Verification items for the finished model (mm, model axes). Face numbers are marked on the shaded views. A direction names the side the tool comes from. Coordinates: 2 decimals unless noted, no trailing zeros. Order: outer loops, then holes, each group sorted by start corner. A loop starts at its lowest first (then second) coordinate and runs counter-clockwise, first axis right, second up. Notation, with made-up numbers: M 1,80.25 L 56,80.25 A22 ccw 56,115.25 Z; hole C 21.25,5 d7. An arc over 180 degrees is marked long. Answer as a JSON object with one key per item and string values. Group by question number.
(1) Access from +Z, -Z, +X, -X, +Y, -Y to the whole of each face (thin tool, end or side, straight path). Record for the marked faces 5 and 6.
(2) Material ranges on line 1 (Z direction, x = 13.1, y = -3.75); line 2 (Z direction, x = -3, y = -6); line 3 (X direction, y = -8.75, z = 31.5), recorded low to high.
(3) Gauge pin test, flat ends, axial feed: pin 1 Ø1.5 at (x, z) = (11, 37) entering from -Y; pin 2 Ø5 at (x, z) = (13.1, 33.2) entering from +Y. Record the tip position at first contact, or that the pin passes through.
(4) Cross-section at A-A (z = 33.2). Enter the section's corners in (x, y).
(5) Cross-section at B-B (y = -1.25). Count the separate pieces of the cut face and the enclosed holes in it, plus the area to 3 significant figures.
(6) Mould release check, pull along X, two halves, no side actions. Record for the marked faces 1, 2, 3 and 4: released by +X, released by -X, zero draft, split by the parting line, or undercut.
(7) Cross-section at D-D (z = 10). Enter the section's corners in (x, y), plus the area to 3 significant figures.
(8) Cross-section at C-C (x = -14). Enter the section's corners in (y, z).
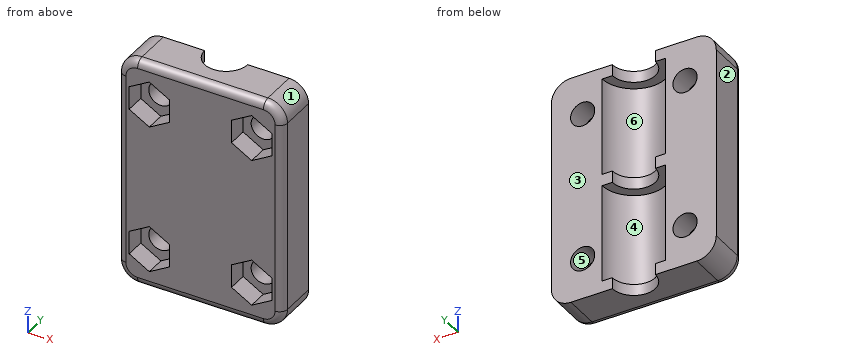
from build123d import *

# Parameters (mm, degrees)
F1_DEPTH = 15.5
F2_DEPTH = 12.6
F3_R     = 3.1
F4_DEPTH = 11.101
F6_R     = 3.1
F7_DEPTH = 5
F9_R     = 5
F10_R    = 2


# Not quite as in the source:
# - a feature names something its author has since deleted; it is built from what else it names


with BuildPart() as f1:
    # F0 (on Top) → F1 (new body, symmetric)
    with BuildSketch(Plane.XY):
        with BuildLine():
            Line((-8.1, 0), (-21.1, 0))
            Line((-21.1, 0), (-21.1, -11.1))
            Line((-21.1, -11.1), (21.1, -11.1))
            Line((21.1, -11.1), (21.1, 0))
            Line((21.1, 0), (8.1, 0))
            ThreePointArc((8.1, 0), (0, -8.1), (-8.1, 0))
        make_face()
        with BuildLine():
            Line((-5.5, 0), (-8.1, 0))
            ThreePointArc((-8.1, 0), (0, -8.1), (8.1, 0))
            Line((8.1, 0), (5.5, 0))
            ThreePointArc((5.5, 0), (0, -5.5), (-5.5, 0))
        make_face()
    extrude(amount=F1_DEPTH, both=True)

    # F0 (on Top) → F2 (cut, symmetric)
    with BuildSketch(Plane.XY):
        with BuildLine():
            Line((-5.5, 0), (-8.1, 0))
            ThreePointArc((-8.1, 0), (0, -8.1), (8.1, 0))
            Line((8.1, 0), (5.5, 0))
            ThreePointArc((5.5, 0), (0, -5.5), (-5.5, 0))
        make_face()
    extrude(amount=F2_DEPTH, both=True, mode=Mode.SUBTRACT)

    # F3 (on Front) → F4 (cut, through all)
    with BuildSketch(Plane.XZ):
        with Locations((13.1, -5)):
            Circle(F3_R)
        with Locations((-13.1, -5)):
            Circle(F3_R)
    extrude(amount=F4_DEPTH, mode=Mode.SUBTRACT)

    # F6 (on face) → F7 (cut)
    with BuildSketch(Plane.XZ.offset(11.1)):
        Polygon((7.95, -2.0266461137), (7.95, -7.9733538863), (13.1, -10.9467077727), (18.25, -7.9733538863), (18.25, -2.0266461137), (13.1, 0.9467077727), align=None)
        with Locations((13.1, -5)):
            Circle(F6_R, mode=Mode.SUBTRACT)
        Polygon((-18.25, -7.9733538863), (-13.1, -10.9467077727), (-7.95, -7.9733538863), (-7.95, -2.0266461137), (-13.1, 0.9467077727), (-18.25, -2.0266461137), align=None)
        with Locations((-13.1, -5)):
            Circle(F6_R, mode=Mode.SUBTRACT)
    extrude(amount=-F7_DEPTH, mode=Mode.SUBTRACT)

    # F8: F1 across plane


with BuildPart() as f1_1:
    add(f1.part)
    add(f1.part.mirror(Plane(origin=(0, -5.9130296111, 14.1), x_dir=(1, 0, 0), z_dir=(0, 0, 1))))

    # F9
    f9_edges = [f1_1.edges().sort_by_distance(p)[0] for p in [
        (21.1, -5.55, 43.7),
        (21.1, -5.55, -15.5),
        (-21.1, -5.55, -15.5),
        (-21.1, -5.55, 43.7),
    ]]
    fillet(f9_edges, radius=F9_R)

    # F10
    f10_edges = [f1_1.edges().sort_by_distance(p)[0] for p in [
        (21.1, -11.1, 14.1),
        (19.635534, -11.1, -14.035534),
        (-21.1, -11.1, 14.1),
        (-19.635534, -11.1, -14.035534),
        (-19.635534, -11.1, 42.235534),
        (0, -11.1, -15.5),
        (0, -11.1, 43.7),
        (19.635534, -11.1, 42.235534),
    ]]
    fillet(f10_edges, radius=F10_R)


solid = f1_1.part
Taken from the geometry:
{
 "1": {"face 5": "+Y, -Y", "face 6": "+Y"},
 "2": {"line 1": "z = -15.5 to -8.1, -1.9 to 30.1, 36.3 to 43.7", "line 2": "z = -15.5 to -12.6, 12.6 to 15.6, 40.8 to 43.7", "line 3": "x = -21.1 to -18.25, -7.95 to 7.95, 18.25 to 21.1"},
 "3": {"pin 1": "stops at y = -6.1", "pin 2": "passes through"},
 "4": {"outline": "M -21.1,-9.1 A2 ccw -19.1,-11.1 L -18.25,-11.1 L -18.25,-6.1 L -16.2,-6.1 L -16.2,0 L -21.1,0 Z; M -10,-6.1 L -7.95,-6.1 L -7.95,-11.1 L 7.95,-11.1 L 7.95,-6.1 L 10,-6.1 L 10,0 L 8.1,0 A8.1 cw -8.1,0 L -10,0 Z; M 16.2,-6.1 L 18.25,-6.1 L 18.25,-11.1 L 19.1,-11.1 A2 ccw 21.1,-9.1 L 21.1,0 L 16.2,0 Z"},
 "5": {"separate pieces": "2", "enclosed holes": "4", "area": "1,460 mm²"},
 "6": {"face 1": "released by +X", "face 2": "released by -X", "face 3": "zero draft", "face 4": "undercut"},
 "7": {"outline": "M -21.1,-9.1 A2 ccw -19.1,-11.1 L 19.1,-11.1 A2 ccw 21.1,-9.1 L 21.1,0 L 8.1,0 A8.1 cw -8.1,0 L -21.1,0 Z", "area": "364 mm²"},
 "8": {"outline": "M -11.1,-13.5 A2 ccw -9.1,-15.5 L 0,-15.5 L 0,-7.97 L -6.1,-7.97 L -6.1,-10.43 L -11.1,-10.43 Z; M -11.1,0.43 L -6.1,0.43 L -6.1,-2.03 L 0,-2.03 L 0,30.23 L -6.1,30.23 L -6.1,27.77 L -11.1,27.77 Z; M -11.1,38.63 L -6.1,38.63 L -6.1,36.17 L 0,36.17 L 0,43.7 L -9.1,43.7 A2 ccw -11.1,41.7 Z"}
}
